Here's how the part is built. I have some questions about the finished solid (model axes, mm). Face numbers are marked on the shaded views. Round coordinates to 2 decimals unless told otherwise and drop trailing zeros. Loops run counter-clockwise (first coordinate to the right, second up) from the corner with the lowest first, then second, coordinate; pieces in that order, holes last. Notation, with made-up numbers: M 67.25,70.25 L 118.25,70.25 A7 cw 118.25,79.25 Z; hole C 43,1 d2. An arc over 180 degrees is marked long. Answer as a JSON object with one key per item and string values.
Autodesk Inventor part; units mm, degrees
ref_plane "YZ Plane" through (0, 0, 0) normal (1, 0, 0) x (0, 1, 0)
ref_plane "XZ Plane" through (0, 0, 0) normal (0, 1, 0) x (-1, 0, 0)
ref_plane "XY Plane" through (0, 0, 0) normal (0, 0, 1) x (1, 0, 0)
sketch "Sketch1" plane through (0, 0, 0) normal (1, 0, 0) x (0, 1, 0)
  circle A0 centre (0, 0) radius 12.5
  line L0 (0, 12.5) -> (0, -12.5)
  line L1 (0, -12.5) -> (12.5, -12.5)
  line L2 (12.5, -12.5) -> (12.5, 12.5)
  line L3 (12.5, 12.5) -> (0, 12.5)
  line L4 (12.5, 12.5) -> (16, 12.5)
  line L5 (16, 12.5) -> (16, -12.5)
  line L6 (16, -12.5) -> (12.5, -12.5)
  line L7 (12.5, -12.5) -> (12.5, 12.5)
  line L8 (16, 12.5) -> (12.5, 12.5)
  line L9 (12.5, 12.5) -> (12.5, 18.5)
  line L10 (12.5, 18.5) -> (16, 18.5)
  line L11 (16, 18.5) -> (16, 12.5)
  line L12 (16, -12.5) -> (12.5, -12.5)
  line L13 (12.5, -12.5) -> (12.5, -18.5)
  line L14 (12.5, -18.5) -> (16, -18.5)
  line L15 (16, -18.5) -> (16, -12.5)
  line L16 (12.5, 18.5) -> (12.5, 12.5)
  line L17 (12.5, -18.5) -> (12.5, -12.5)
  line L18 (16, 18.5) -> (0.5, 18.5)
  line L19 (0.5, 18.5) -> (0.5, 12.5)
  line L20 (0.5, 12.5) -> (16, 12.5)
  line L21 (16, 12.5) -> (16, 18.5)
  line L22 (16, -12.5) -> (0.5, -12.5)
  line L23 (0.5, -12.5) -> (0.5, -18.5)
  line L24 (0.5, -18.5) -> (16, -18.5)
  line L25 (16, -18.5) -> (16, -12.5)
  point P0 (12.5, 0)
  dimension "d0" = 25
  dimension "d1" = 3.5
  dimension "d2" = 25
  dimension "d3" = 6
  dimension "d4" = 6
  dimension "d15" = 15.5
  dimension "d16" = 15.5
extrude "Extrusion3" add sketch "Sketch1" along normal blind 5 contours L2 L1 A0 | L2 L4 L5 L6 | A0 L3 L2 | L13 L24 L23 L1 | L6 L15 L14 L13 | L9 L10 L11 L4 | L3 L19 L18 L9
sketch "Sketch4" plane through (0, 16, 18.5) normal (0, 1, 0) x (1, 0, 0)
  line L0 (0, 37) -> (5, 37)
  line L1 (0, 0) -> (5, 0)
  circle A0 centre (2.5, 2.879) radius 1.5875
  circle A1 centre (2.5, 34.121) radius 1.5875
  line L2 (0, 37) -> (0, 0)
  line L3 (5, 37) -> (5, 0)
  line L4 (0, 18.5) -> (5, 18.5)
  dimension "d23" = 3.175
  dimension "d24" = 3.175
  dimension "d27" = 2.5
  dimension "d28" = 15.621
  dimension "d29" = 15.621
extrude "Extrusion5" cut sketch "Sketch4" against normal blind 20 contours A0 | A1
properties part number "TubeClamp"
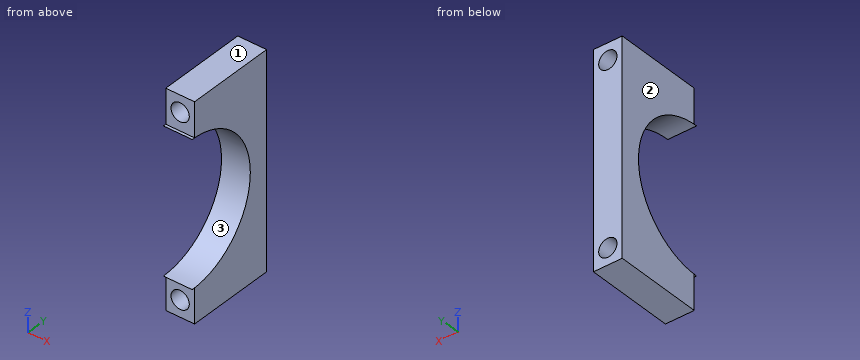
Item 1: I want a section at C-C on y = 7.25. List the corners of the cut face in (x, z) for me (1 decimal), plus the area to 3 significant figures.
Solution:
{"outline": "M 0,-18.5 L 5,-18.5 L 5,-10.2 L 0,-10.2 Z; M 0,10.2 L 5,10.2 L 5,18.5 L 0,18.5 Z; hole C 2.5,-15.6 d3.2; hole C 2.5,15.6 d3.2", "area": "67.3 mm2"}
Item 2: If I drill on L1, parallel to Z at x = 2.5, y = 5.5; L2, parallel to Z at x = 2.1, y = 6.5; L3, parallel to Z at x = 3.65, y = 13.5, over which ranges is the centre line in solid material (lowest first)? Write a range as from..to.
Solution:
{"L1": "z = -18.5..-17.21, -14.03..-11.22, 11.22..14.03, 17.21..18.5", "L2": "z = -18.5..-17.16, -14.08..-10.68, 10.68..14.08, 17.16..18.5", "L3": "z = -18.5..-16.72, -14.53..14.53, 16.72..18.5"}
Item 3: I want a section at B-B on x = 2.5. List the corners of the cut face in (y, z) for me.
Solution:
{"outline": "M 0,-12.5 L 0.5,-12.5 L 0.5,-14.03 L 16,-14.03 L 16,14.03 L 0.5,14.03 L 0.5,12.5 L 0,12.5 A12.5 cw Z; M 0.5,-18.5 L 16,-18.5 L 16,-17.21 L 0.5,-17.21 Z; M 0.5,17.21 L 16,17.21 L 16,18.5 L 0.5,18.5 Z"}
Item 4: I want a section at D-D on x = 0.45. List the corners of the cut face in (y, z) for me.
Solution:
{"outline": "M 0,-12.5 L 0.5,-12.5 L 0.5,-18.5 L 16,-18.5 L 16,18.5 L 0.5,18.5 L 0.5,12.5 L 0,12.5 A12.5 cw Z"}
Item 5: We'd pull the mould along Z, two halves only. Please class the marked faces 1, 2 and 3: +Z half, -Z half, draft (parallel to the pull), parting line (faces both ways), or undercut.
Solution:
{"face 1": "+Z half", "face 2": "draft", "face 3": "undercut"}
Item 6: For P1, Ø1.5, axis at y = 11, z = -5, coming from the -X side; P2, Ø1.5, axis at y = 5, z = 9.5, coming from the -X side, each with a flat end and sliding along its axis, tell me the tip position at first contact or that it passes through.
Solution:
{"P1": "stops at x = 0", "P2": "passes through"}
Item 7: I want a section at A-A on y = 11. List the corners of the cut face in (x, z) for me (1 decimal).
Solution:
{"outline": "M 0,-18.5 L 5,-18.5 L 5,-5.9 L 0,-5.9 Z; M 0,5.9 L 5,5.9 L 5,18.5 L 0,18.5 Z; hole C 2.5,-15.6 d3.2; hole C 2.5,15.6 d3.2"}
